```python
from build123d import *

# Parameters (mm, degrees)
F0_R     = 7
F1_DEPTH = 7
F2_R     = 10
F2_R_2   = 8.5
F2_R_3   = 7
F3_DEPTH = 3.5
F4_R     = 10
F4_R_2   = 8.5
F5_DEPTH = 8


with BuildPart() as f1:
    # F0 (on Top) → F1 (new body)
    with BuildSketch(Plane.XY):
        Circle(F0_R)
        with BuildLine():
            ThreePointArc((-4.2426406871, 1.5), (0, 4.5), (4.2426406871, 1.5))
            Line((4.2426406871, 1.5), (6, 1.5))
            Line((6, 1.5), (6, 0))
            Line((6, 0), (6, -1.5))
            Line((6, -1.5), (4.2426406871, -1.5))
            ThreePointArc((4.2426406871, -1.5), (0, -4.5), (-4.2426406871, -1.5))
            Line((-4.2426406871, -1.5), (-6, -1.5))
            Line((-6, -1.5), (-6, 0))
            Line((-6, 0), (-6, 1.5))
            Line((-6, 1.5), (-4.2426406871, 1.5))
        make_face(mode=Mode.SUBTRACT)
    extrude(amount=F1_DEPTH)

    # F2 (on face) → F3 (join)
    with BuildSketch(Plane.XY.offset(7)):
        Circle(F2_R)
        Circle(F2_R_2, mode=Mode.SUBTRACT)
        Circle(F2_R_2)
        Circle(F2_R_3, mode=Mode.SUBTRACT)
        Circle(F2_R_3)
        with BuildLine():
            Line((-6, 1.5), (-4.2426406871, 1.5))
            ThreePointArc((-4.2426406871, 1.5), (0, 4.5), (4.2426406871, 1.5))
            Line((4.2426406871, 1.5), (6, 1.5))
            Line((6, 1.5), (6, -1.5))
            Line((6, -1.5), (4.2426406871, -1.5))
            ThreePointArc((4.2426406871, -1.5), (0, -4.5), (-4.2426406871, -1.5))
            Line((-4.2426406871, -1.5), (-6, -1.5))
            Line((-6, -1.5), (-6, 1.5))
        make_face(mode=Mode.SUBTRACT)
        with BuildLine():
            ThreePointArc((4.2426406871, 1.5), (0, 4.5), (-4.2426406871, 1.5))
            Line((-4.2426406871, 1.5), (-6, 1.5))
            Line((-6, 1.5), (-6, -1.5))
            Line((-6, -1.5), (-4.2426406871, -1.5))
            ThreePointArc((-4.2426406871, -1.5), (0, -4.5), (4.2426406871, -1.5))
            Line((4.2426406871, -1.5), (6, -1.5))
            Line((6, -1.5), (6, 1.5))
            Line((6, 1.5), (4.2426406871, 1.5))
        make_face()
    extrude(amount=F3_DEPTH)

    # F4 (on face) → F5 (join)
    with BuildSketch(Plane.XY.offset(10.5)):
        Circle(F4_R)
        Circle(F4_R_2, mode=Mode.SUBTRACT)
    extrude(amount=F5_DEPTH)


solid = f1.part
```
Check sheet for the modelled part. Datum: model origin and axes. Units: mm. A direction names the side the tool comes from. Round coordinates to 2 decimals unless told otherwise and drop trailing zeros. Loops run counter-clockwise (first coordinate to the right, second up) from the corner with the lowest first, then second, coordinate; pieces in that order, holes last. Notation, with made-up numbers: M 32.5,12 L 91.5,12 A20 ccw 91.5,47 Z; hole C 40,34 d10. An arc over 180 degrees is marked long. Answer as a JSON object with one key per item and string values.
1. Section check A-A (z = 3). Record the boundary of the cut face in (x, y), plus the area to 3 significant figures.
Reply:
{"outline": "C 0,0 d14; hole M -6,-1.5 L -4.24,-1.5 A4.5 ccw 4.24,-1.5 L 6,-1.5 L 6,1.5 L 4.24,1.5 A4.5 ccw -4.24,1.5 L -6,1.5 Z", "area": "80.8 mm²"}
2. Section check C-C (x = 0). Record the boundary of the cut face in (y, z), plus the area to 3 significant figures.
Reply:
{"outline": "M -10,7 L -7,7 L -7,0 L -4.5,0 L -4.5,7 L 4.5,7 L 4.5,0 L 7,0 L 7,7 L 10,7 L 10,18.5 L 8.5,18.5 L 8.5,10.5 L -8.5,10.5 L -8.5,18.5 L -10,18.5 Z", "area": "129 mm²"}
3. Scan lines: line 1 (Y direction, x = 0, z = 13.5); line 2 (Z direction, x = 0.5, y = 6); line 3 (Z direction, x = 2, y = 8.5). Record each from-to range of solid material in increasing order.
Reply:
{"line 1": "y = -10 to -8.5, 8.5 to 10", "line 2": "z = 0 to 10.5", "line 3": "z = 7 to 18.5"}
4. Section check B-B (y = 0). Record the boundary of the cut face in (x, z).
Reply:
{"outline": "M -10,7 L -7,7 L -7,0 L -6,0 L -6,7 L 6,7 L 6,0 L 7,0 L 7,7 L 10,7 L 10,18.5 L 8.5,18.5 L 8.5,10.5 L -8.5,10.5 L -8.5,18.5 L -10,18.5 Z"}
5. Gauge pin test, flat ends, axial feed: P1, Ø5, axis at x = 3.5, y = -6.5, coming from the -Z side; P2, Ø8.5, axis at x = 3, y = -1.5, coming from the +Z side; P3, Ø1.9, axis at x = 5, z = 4, coming from the +Y side; P4, Ø0.9, axis at y = 0.5, z = 2, coming from the -X side. Record the tip position at first contact, or that the pin passes through.
Reply:
{"P1": "stops at z = 0", "P2": "stops at z = 10.5", "P3": "stops at y = 5.71", "P4": "stops at x = -7"}
6. Section check D-D (x = 8). Record the boundary of the cut face in (y, z).
Reply:
{"outline": "M -6,7 L 6,7 L 6,18.5 L 2.87,18.5 L 2.87,10.5 L -2.87,10.5 L -2.87,18.5 L -6,18.5 Z"}
7. Mould release check, pull along Y, two halves, no side actions. Record for faces 4 (the flat face through (-4.5, -7.4, 18.5)), 5 (the flat face through (0, 0, 10.5)), 6 (the flat face through (-5, 1.5, 3)), 7 (the cylindrical face through (6.466, -2.681, 3.451)): pulls with the +Y half, pulls with the -Y half, needs draft (parallel to the pull), parting line crosses it, or undercut.
Reply:
{"face 4": "needs draft", "face 5": "undercut", "face 6": "undercut", "face 7": "parting line crosses it"}
8. Access from +Z, -Z, +X, -X, +Y, -Y to the whole of each face (thin tool, end or side, straight path). Record for faces 1 (the cylindrical face through (4.57, 7.167, 14.444)), 2 (the cylindrical face through (0.1, -4.5, 3.5)), 3 (the flat face through (0, -5, 0)).
Reply:
{"face 1": "+Z", "face 2": "-Z", "face 3": "-Z, +X, -X, +Y, -Y"}
